```python
from build123d import *

# Parameters (mm, degrees)
SKETCH1_R           = 2.55
SKETCH1_R_2         = 2
BOSS_EXTRUDE1_DEPTH = 5


with BuildPart() as part:
    # Sketch1 → Boss-Extrude1 (new body)
    with BuildSketch(Plane.XY):
        Polygon((-35, -12.5), (-35, -52.5), (35, -52.5), (35, -12.5), (35, 12.5), (-35, 12.5), align=None)
        with Locations((-25, -22.5)):
            Circle(SKETCH1_R, mode=Mode.SUBTRACT)
        with Locations((-25, -42.5)):
            Circle(SKETCH1_R, mode=Mode.SUBTRACT)
        with Locations((25, -42.5)):
            Circle(SKETCH1_R, mode=Mode.SUBTRACT)
        with Locations((25, -22.5)):
            Circle(SKETCH1_R, mode=Mode.SUBTRACT)
        with Locations((-12.5, 0)):
            Circle(SKETCH1_R_2, mode=Mode.SUBTRACT)
        with Locations((12.5, 0)):
            Circle(SKETCH1_R_2, mode=Mode.SUBTRACT)
    extrude(amount=BOSS_EXTRUDE1_DEPTH)


solid = part.part
```
Can you work these out from the model? Positions are in its coordinate system, mm. Round coordinates to 2 decimals unless told otherwise and drop trailing zeros. Loops run counter-clockwise (first coordinate to the right, second up) from the corner with the lowest first, then second, coordinate; pieces in that order, holes last. Notation, with made-up numbers: M 57.25,73.5 L 87.25,73.5 A38 ccw 87.25,111.5 Z; hole C -25.5,-21.5 d8. An arc over 180 degrees is marked long. Write item = value, one per line. Start each with the question number.
(1) I'm going to push a flat-ended pin straight in: P1, Ø4, axis at x = -25, y = -22.5, coming from the +Z side. Where does the tip first touch, or does it pass through?
(2) Suppose I cut it at A-A on x = -25. Write out the boundary of the cut face in (y, z), plus the area to 3 significant figures.
(3) Suppose I cut it at C-C on y = -42.5. Write out the boundary of the cut face in (x, z), plus the area to 3 significant figures.
(4) If we mould it in two halves opening along X, with no side actions, what happens to faces 1 (the face through (35, -20, 2)), 2 (the face through (0, -52.5, 2)), 3 (the face through (-14.1, -1.2, 2.5))? For each: released by +X, released by -X, zero draft, split by the parting line, or undercut.
(5) Suppose I cut it at B-B on z = 3.1. Write out the boundary of the cut face in (x, y).
(6) Suppose I cut it at D-D on x = -12.5. Write out the boundary of the cut face in (y, z), plus the area to 3 significant figures.
(7) I need wall thicknesses on line 1 along Y through (x, z) = (25, 3.55); line 2 along Y through (x, z) = (-12.5, 3.45); line 3 along Y through (x, z) = (27, 0.45). Which ranges of each line are inside material? Lowest first, please.
Answer block:
q1.P1 = through
q2.outline = M -52.5,0 L -45.05,0 L -45.05,5 L -52.5,5 Z; M -39.95,0 L -25.05,0 L -25.05,5 L -39.95,5 Z; M -19.95,0 L 12.5,0 L 12.5,5 L -19.95,5 Z
q2.area = 274 mm²
q3.outline = M -35,0 L -27.55,0 L -27.55,5 L -35,5 Z; M -22.45,0 L 22.45,0 L 22.45,5 L -22.45,5 Z; M 27.55,0 L 35,0 L 35,5 L 27.55,5 Z
q3.area = 299 mm²
q4.face_1 = released by +X
q4.face_2 = zero draft
q4.face_3 = undercut
q5.outline = M -35,-52.5 L 35,-52.5 L 35,12.5 L -35,12.5 Z; hole C -25,-42.5 d5.1; hole C -25,-22.5 d5.1; hole C -12.5,0 d4; hole C 12.5,0 d4; hole C 25,-42.5 d5.1; hole C 25,-22.5 d5.1
q6.outline = M -52.5,0 L -2,0 L -2,5 L -52.5,5 Z; M 2,0 L 12.5,0 L 12.5,5 L 2,5 Z
q6.area = 305 mm²
q7.line_1 = -52.5 to -45.05, -39.95 to -25.05, -19.95 to 12.5
q7.line_2 = -52.5 to -2, 2 to 12.5
q7.line_3 = -52.5 to -44.08, -40.92 to -24.08, -20.92 to 12.5
